from build123d import *

# Parameters (mm, degrees)
MODEL_R         = 1.15
MODEL_R_2       = 1.5
EXTRUDE_1_DEPTH = 2


with BuildPart() as part:
    # Model → Бобышка-Вытянуть1 (new body)
    # profile 1 of 3: a face of its own
    with BuildSketch(Plane.XY):
        with BuildLine():
            ThreePointArc((-11, 0), (-14.807611845, 9.192388155), (-24, 13))
            ThreePointArc((-24, 13), (-28.725958264, 12.110545755), (-32.805220584, 9.563895152))
            ThreePointArc((-32.805220584, 9.563895152), (-36.734496712, -2.613923009), (-28.325743505, -12.259198307))
            ThreePointArc((-28.325743505, -12.259198307), (-26.194358905, -12.813461242), (-24, -13))
            ThreePointArc((-24, -13), (-14.807611845, -9.192388155), (-11, 0))
        make_face()
        with Locations((-24, 0)):
            Circle(MODEL_R, mode=Mode.SUBTRACT)
    # profile 2 of 3: a face of its own
    with BuildSketch(Plane.XY):
        with BuildLine():
            ThreePointArc((-28.325743505, -12.259198307), (-36.734496712, -2.613923009), (-32.805220584, 9.563895152))
            Line((-32.805220584, 9.563895152), (-45.031973981, -1.692947273))
            ThreePointArc((-45.031973981, -1.692947273), (-45.93873001, -4.503213002), (-43.998248501, -6.729045763))
            Line((-43.998248501, -6.729045763), (-28.325743505, -12.259198307))
        make_face()
        with Locations((-43, -3.9)):
            Circle(MODEL_R, mode=Mode.SUBTRACT)
    # profile 3 of 3: a face of its own
    with BuildSketch(Plane.XY):
        with BuildLine():
            Line((-10, 18), (-15, 18))
            ThreePointArc((-15, 18), (-16.464466094, 14.464466094), (-20, 13))
            Line((-20, 13), (-24, 13))
            ThreePointArc((-24, 13), (-14.807611845, 9.192388155), (-11, 0))
            ThreePointArc((-11, 0), (-14.807611845, -9.192388155), (-24, -13))
            Line((-24, -13), (-20, -13))
            ThreePointArc((-20, -13), (-16.464466094, -14.464466094), (-15, -18))
            Line((-15, -18), (-10, -18))
            Line((-10, -18), (-10, -15))
            Line((-10, -15), (-5, -15))
            Line((-5, -15), (-5, -18))
            Line((-5, -18), (5, -18))
            Line((5, -18), (5, -15))
            Line((5, -15), (10, -15))
            Line((10, -15), (10, -18))
            Line((10, -18), (15, -18))
            ThreePointArc((15, -18), (16.464466094, -14.464466094), (20, -13))
            Line((20, -13), (24, -13))
            ThreePointArc((24, -13), (26.194358905, -12.813461242), (28.325743505, -12.259198307))
            Line((28.325743505, -12.259198307), (43.998248501, -6.729045763))
            ThreePointArc((43.998248501, -6.729045763), (45.93873001, -4.503213002), (45.031973981, -1.692947273))
            Line((45.031973981, -1.692947273), (32.805220584, 9.563895152))
            ThreePointArc((32.805220584, 9.563895152), (28.725958264, 12.110545755), (24, 13))
            Line((24, 13), (20, 13))
            ThreePointArc((20, 13), (16.464466094, 14.464466094), (15, 18))
            Line((15, 18), (10, 18))
            Line((10, 18), (10, 15))
            Line((10, 15), (5, 15))
            Line((5, 15), (5, 18))
            Line((5, 18), (-5, 18))
            Line((-5, 18), (-5, 15))
            Line((-5, 15), (-10, 15))
            Line((-10, 15), (-10, 18))
        make_face()
        with Locations((43, -3.9)):
            Circle(MODEL_R, mode=Mode.SUBTRACT)
        Circle(MODEL_R_2, mode=Mode.SUBTRACT)
        with Locations((24, 0)):
            Circle(MODEL_R, mode=Mode.SUBTRACT)
    extrude(amount=EXTRUDE_1_DEPTH)


solid = part.part
Could you check a few things on this model? Use its own coordinates, in mm. A direction names the side the tool comes from. Round coordinates to 2 decimals unless told otherwise and drop trailing zeros. Order: outer loops, then holes, each group sorted by start corner. A loop starts at its lowest first (then second) coordinate and runs counter-clockwise, first axis right, second up.
(1) If we mould it in two halves opening along X, with no side actions, what happens to faces 1 (the flat face through (-12, 18, 1)), 2 (the flat face through (-36.272, -9.455, 0.986)), 3 (the flat face through (5, 16, 1))? For each: released by +X, released by -X, zero draft, split by the parting line, or undercut.
Response values:
face 1: zero draft
face 2: released by -X
face 3: undercut
(2) I'm going to push flat-ended pins straight in: pin 1 (0.6 mm diameter, centred on x = -21.5, z = 0.5, fed in from -Y); pin 2 (0.6 mm diameter, centred on x = -7.5, z = 0.5, fed in from -Y). Where does each tip first touch, or does it pass through?
Response values:
pin 1: stops at y = -13
pin 2: stops at y = -15
(3) Imagine slicing it at A-A (y = -3.9). Write out the boundary of the cut face in (x, z), plus the area to 3 significant figures.
Response values:
outline: (-46, 0) - (-44.15, 0) - (-44.15, 2) - (-46, 2) - close; (-41.85, 0) - (41.85, 0) - (41.85, 2) - (-41.85, 2) - close; (44.15, 0) - (46, 0) - (46, 2) - (44.15, 2) - close
area: 175 mm2
(4) Imagine slicing it at D-D (z = 1.55). Count the separate pieces of the cut face and the enclosed holes in it, plus the area to 3 significant figures.
Response values:
separate pieces: 1
enclosed holes: 5
area: 2,220 mm2
(5) Imagine slicing it at C-C (y = 0). Write out the boundary of the cut face in (x, z).
Response values:
outline: (-43.19, 0) - (-25.15, 0) - (-25.15, 2) - (-43.19, 2) - close; (-22.85, 0) - (-1.5, 0) - (-1.5, 2) - (-22.85, 2) - close; (1.5, 0) - (22.85, 0) - (22.85, 2) - (1.5, 2) - close; (25.15, 0) - (43.19, 0) - (43.19, 2) - (25.15, 2) - close
(6) Imagine slicing it at B-B (x = 0). Write out the boundary of the cut face in (y, z), plus the area to 3 significant figures.
Response values:
outline: (-18, 0) - (-1.5, 0) - (-1.5, 2) - (-18, 2) - close; (1.5, 0) - (18, 0) - (18, 2) - (1.5, 2) - close
area: 66.0 mm2
(7) Which directions (+Z, -Z, +X, -X, +Y, -Y) give clear straight access to the entire face, cutting with the end or side of a thin tool? Please do faces 4 (the flat face through (-5, -16, 1)), 5 (the flat face through (-22, -13, 1)), 6 (the flat face through (22, -13, 1)), 7 (the flat face through (-10, 16, 1)).
Response values:
face 4: +Z, -Z, -Y
face 5: +Z, -Z, -X, -Y
face 6: +Z, -Z, +X, -Y
face 7: +Z, -Z, +Y
(8) Please list where these lines run through material, in increasing order: line 1 along X through (y, z) = (-3.5, 1.8); line 2 along Y through (x, z) = (0, 1.35); line 3 along Y through (x, z) = (24, 1.65).
Response values:
line 1: x = -45.97 to -44.08, -41.92 to 41.92, 44.08 to 45.97
line 2: y = -18 to -1.5, 1.5 to 18
line 3: y = -13 to -1.15, 1.15 to 13
